from build123d import *

# Parameters (mm, degrees)
EXTRUDE_1_DEPTH     = 2
EXTRUDE_START       = -2
EXTRUDE_6_DEPTH     = 2
SKETCH_3_R          = 1.45
CUT_EXTRUDE_1_DEPTH = 2


with BuildPart() as part:
    # 草图1 → 凸台-拉伸1 (new body)
    with BuildSketch(Plane.XY):
        with BuildLine():
            ThreePointArc((34.999399669, -35.707730574), (0, -50), (-34.999399669, -35.707730574))
            ThreePointArc((-34.999399669, -35.707730574), (-40.655970089, -35.764397047), (-40.599303617, -41.420967466))
            ThreePointArc((-40.599303617, -41.420967466), (0, -58), (40.599303617, -41.420967466))
            ThreePointArc((40.599303617, -41.420967466), (40.655970089, -35.764397047), (34.999399669, -35.707730574))
        make_face()
    extrude(amount=EXTRUDE_1_DEPTH)

    # 草图2 → 凸台-拉伸6 (add)
    with BuildSketch(Plane.XY.offset(2).offset(EXTRUDE_START)):
        with BuildLine():
            add(Edge.make_bspline(
                [(-34.999399669, -35.707730574), (-31.293036679, -34.051470167), (-32.304776642, -38.162827543)],
                knots=[0, 0, 0, 1, 1, 1], degree=2))
            ThreePointArc((-34.999399669, -35.707730574), (-33.674469744, -36.959844257), (-32.304776642, -38.162827543))
        make_face()
        with BuildLine():
            add(Edge.make_bspline(
                [(-29.427336681, -40.423159895), (-26.001624486, -38.244898865), (-26.403964274, -42.459753539)],
                knots=[0, 0, 0, 1, 1, 1], degree=2))
            ThreePointArc((-29.427336681, -40.423159895), (-27.934216832, -41.469018918), (-26.403964274, -42.459753539))
        make_face()
        with BuildLine():
            add(Edge.make_bspline(
                [(-23.228081101, -44.277039743), (-20.15603281, -41.623203943), (-19.940397248, -45.851723605)],
                knots=[0, 0, 0, 1, 1, 1], degree=2))
            ThreePointArc((-23.228081101, -44.277039743), (-21.598594585, -45.094353437), (-19.940397248, -45.851723605))
        make_face()
        with BuildLine():
            add(Edge.make_bspline(
                [(-16.5337593, -47.18723136), (-13.880850288, -44.114382693), (-13.051835275, -48.266443788)],
                knots=[0, 0, 0, 1, 1, 1], degree=2))
            ThreePointArc((-16.5337593, -47.18723136), (-14.802635794, -47.758580104), (-13.051835275, -48.266443788))
        make_face()
        with BuildLine():
            add(Edge.make_bspline(
                [(-9.487049125, -49.091709065), (-7.309821542, -45.665339966), (-5.885096092, -49.65244852)],
                knots=[0, 0, 0, 1, 1, 1], degree=2))
            ThreePointArc((-9.487049125, -49.091709065), (-7.69118452, -49.404915552), (-5.885096092, -49.65244852))
        make_face()
        with BuildLine():
            add(Edge.make_bspline(
                [(-2.238138968, -49.949882222), (-0.58299664, -46.243019798), (1.407073696, -49.980197515)],
                knots=[0, 0, 0, 1, 1, 1], degree=2))
            ThreePointArc((-2.238138968, -49.949882222), (-0.415809002, -49.998270999), (1.407073696, -49.980197515))
        make_face()
        with BuildLine():
            add(Edge.make_bspline(
                [(5.058473235, -49.743460359), (6.156253823, -45.835109949), (8.669254151, -49.242705373)],
                knots=[0, 0, 0, 1, 1, 1], degree=2))
            ThreePointArc((5.058473235, -49.743460359), (6.868428764, -49.526000104), (8.669254151, -49.242705373))
        make_face()
        with BuildLine():
            add(Edge.make_bspline(
                [(31.66559238, -38.694835046), (30.424637319, -34.829559417), (34.400675338, -36.284894051)],
                knots=[0, 0, 0, 1, 1, 1], degree=2))
            ThreePointArc((31.66559238, -38.694835046), (33.055103788, -37.514798594), (34.400675338, -36.284894051))
        make_face()
        with BuildLine():
            add(Edge.make_bspline(
                [(25.69413065, -42.893025659), (25.029188635, -38.888256343), (28.750957058, -40.906997791)],
                knots=[0, 0, 0, 1, 1, 1], degree=2))
            ThreePointArc((25.69413065, -42.893025659), (27.240649231, -41.927878905), (28.750957058, -40.906997791))
        make_face()
        with BuildLine():
            add(Edge.make_bspline(
                [(19.175043133, -46.177025899), (19.100286249, -42.118117602), (22.488462044, -44.657239893)],
                knots=[0, 0, 0, 1, 1, 1], degree=2))
            ThreePointArc((19.175043133, -46.177025899), (20.84560753, -45.44733927), (22.488462044, -44.657239893))
        make_face()
        with BuildLine():
            add(Edge.make_bspline(
                [(12.247272863, -48.476843002), (12.764294423, -44.450304307), (15.746664505, -47.455690459)],
                knots=[0, 0, 0, 1, 1, 1], degree=2))
            ThreePointArc((12.247272863, -48.476843002), (14.006277895, -47.998168502), (15.746664505, -47.455690459))
        make_face()
    extrude(amount=EXTRUDE_6_DEPTH)

    # 草图3 → 切除-拉伸1 (cut)
    with BuildSketch(Plane.XY.offset(2)):
        with Locations((-37.799351643, -38.56434902)):
            Circle(SKETCH_3_R)
        with Locations((0.328913231, -53.956500006)):
            Circle(SKETCH_3_R)
        with Locations((37.799351643, -38.56434902)):
            Circle(SKETCH_3_R)
    extrude(amount=-CUT_EXTRUDE_1_DEPTH, mode=Mode.SUBTRACT)


solid = part.part
Check sheet for the modelled part. Datum: model origin and axes. Units: mm. A direction names the side the tool comes from. Round coordinates to 2 decimals unless told otherwise and drop trailing zeros. Loops run counter-clockwise (first coordinate to the right, second up) from the corner with the lowest first, then second, coordinate; pieces in that order, holes last. Notation, with made-up numbers: (10.25, 23) -> (66.25, 23) arc R19 cw to (66.25, 54) -> close; hole circle Ø1 at (25, -20.75). An arc over 180 degrees is marked (long way). Put each result on its own line as item: value. Start each with the question number.
1. Scan lines: probe 1 along X at (y, z) = (-38, 0.9); probe 2 along X at (y, z) = (-37.75, 1.7); probe 3 along X at (y, z) = (-45.75, 0.1). Record each from-to range of solid material in increasing order.
2. Access from +Z, -Z, +X, -X, +Y, -Y to the whole of each face (thin tool, end or side, straight path). Record for faces 4 (the face through (0, -50, 2)), 5 (the face through (-4.039, -49.837, 0.986)).
3. Section check C-C (x = 29.5). Enter the section's corners in (y, z).
4. Section check A-A (z = 1.45). Give the number of separate pieces and of enclosed holes in the cut face, plus the area to 3 significant figures.
5. Gauge pin test, flat ends, axial feed: pin 1 (1.7 mm diameter, centred on x = 0.33, y = -53.96, fed in from -Z); pin 2 (3.5 mm diameter, centred on x = -37.8, y = -38.56, fed in from +Z). Record the tip position at first contact, or that the pin passes through.
6. Draft check along X on faces 1 (the face through (0, -50, 0)), 2 (the face through (-0.63, -57.997, 0.986)), 3 (the face through (0.14, -52.52, 1.01)). Enter one of: +X half, -X half, draft (parallel to the pull), parting line (faces both ways), or undercut.
7. Section check B-B (x = 18). Enter the section's corners in (y, z).
Findings:
1. probe 1: x = -41.76 to -39.14, -36.46 to -32.27, 31.48 to 36.46, 39.14 to 41.76
1. probe 2: x = -41.72 to -39, -36.6 to -32.21, 31.43 to 36.6, 39 to 41.72
1. probe 3: x = -35.65 to -19.95, 19.18 to 35.65
2. face 4: +Z, +X, -X, +Y, -Y
2. face 5: +Z, -Z, +Y
3. outline: (-49.94, 0) -> (-40.37, 0) -> (-40.37, 2) -> (-49.94, 2) -> close
4. separate pieces: 1
4. enclosed holes: 3
4. area: 751 mm^2
5. pin 1: passes through
5. pin 2: stops at z = 2
6. face 1: draft
6. face 2: parting line
6. face 3: undercut
7. outline: (-55.14, 0) -> (-46.65, 0) -> (-46.65, 2) -> (-55.14, 2) -> close
